Here's how the part is built. I have some questions about the finished solid (model axes, mm). A direction names the side the tool comes from. Coordinates: 2 decimals unless noted, no trailing zeros. Write each loop counter-clockwise with the first axis right and the second up, starting at its lowest first coordinate (ties: lowest second). Pieces come first, ordered by that corner, then holes. Notation, with made-up numbers: M -7,31.25 L 49,31.25 A19 cw 49,62.25 Z; hole C 65,87 d10. An arc over 180 degrees is marked long. Use one line per item in the form item = value. Start each with the question number.
1. Thinking about a two-plate mould opening in Y: for faces 1 (the face through (1, 0, 39)), 2 (the face through (1, 56, 80)), 3 (the face through (0.99, 93.74, 42.34)), which applies, released by +Y, released by -Y, zero draft, split by the parting line, or undercut?
2. On a 3-axis mill with a long thin cutter (end or side, diameter ignored), from which of +Z, -Z, +X, -X, +Y, -Y can I reach the whole of each face in a straight line? I mean faces 4 (the face through (0, 54, 39)), 5 (the face through (2, 54, 33)). Say none if no direction works.
3. I want a section at D-D, the plane z = 69.5. List the corners of the cut face in (x, y) for me, plus the area to 3 significant figures.
4. I want a section at C-C, the plane x = 1.2. Count the separate pieces of the cut face and the enclosed holes in it, plus the area to 3 significant figures.
5. I want a section at B-B, the plane z = 20. List the corners of the cut face in (x, y) for me, plus the area to 3 significant figures.
6. Please list where these lines run through material, in increasing order: line 1 along Y through (x, z) = (1.05, 20); line 2 along Z through (x, y) = (1.35, 92.5); line 3 along Y through (x, z) = (1.35, 73.5). Write a range as [from, to].
7. I'm going to push flat-ended pins straight in: pin 1 Ø3 at (y, z) = (40, 20) entering from -X; pin 2 Ø2 at (y, z) = (55, 28) entering from -X; pin 3 Ø6 at (y, z) = (56.5, 34) entering from +X. Where does each tip first touch, or does it pass through?
8. I want a section at A-A, the plane y = 55. List the corners of the cut face in (x, z) for me, plus the area to 3 significant figures.
from build123d import *

# Parameters (mm, degrees)
SKETCH1_W           = 155
SKETCH1_H           = 110
BOSS_EXTRUDE1_DEPTH = 80
SKETCH2_W           = 151
SKETCH2_H           = 106
CUT_EXTRUDE1_DEPTH  = 78
SKETCH3_R           = 2.5
CUT_EXTRUDE2_DEPTH  = 2
SKETCH7_R           = 1.6
CUT_EXTRUDE7_DEPTH  = 2
SKETCH4_W           = 27.5
SKETCH4_H           = 46.8
CUT_EXTRUDE8_DEPTH  = 2
SKETCH8_W           = 4
SKETCH8_H           = 53
CUT_EXTRUDE9_DEPTH  = 2
SKETCH9_W           = 14
SKETCH9_H           = 14
CUT_EXTRUDE10_DEPTH = 2
SKETCH10_W          = 25.2
SKETCH10_H          = 71.2
SKETCH10_R          = 1.25
CUT_EXTRUDE12_DEPTH = 2
SKETCH11_R          = 2.5
SKETCH11_R_2        = 4.5
CUT_EXTRUDE13_DEPTH = 2
SKETCH12_W          = 152.88518354
SKETCH12_H          = 110
CUT_EXTRUDE14_DEPTH = 80


with BuildPart() as part:
    # Sketch1 → Boss-Extrude1 (new body)
    with BuildSketch(Plane.XY):
        with Locations((77.5, 55)):
            Rectangle(SKETCH1_W, SKETCH1_H)
    extrude(amount=BOSS_EXTRUDE1_DEPTH)

    # Sketch2 → Cut-Extrude1 (cut)
    with BuildSketch(Plane.XY.offset(80)):
        with Locations((77.5, 55)):
            Rectangle(SKETCH2_W, SKETCH2_H)
    extrude(amount=-CUT_EXTRUDE1_DEPTH, mode=Mode.SUBTRACT)

    # Sketch3 → Cut-Extrude2 (cut)
    with BuildSketch(Plane.XY.offset(2)):
        with Locations((145, 100.5)):
            Circle(SKETCH3_R)
        with Locations((145, 9.5)):
            Circle(SKETCH3_R)
        with Locations((10, 9.5)):
            Circle(SKETCH3_R)
        with Locations((10, 100.5)):
            Circle(SKETCH3_R)
    extrude(amount=-CUT_EXTRUDE2_DEPTH, mode=Mode.SUBTRACT)

    # Sketch7 → Cut-Extrude7 (cut)
    with BuildSketch(Plane(origin=(0, 110, 0), x_dir=(1, 0, 0), z_dir=(0, 1, 0))):
        with Locations((44.48, -20.14450396)):
            Circle(SKETCH7_R)
        with Locations((95.28, -17.14)):
            Circle(SKETCH7_R)
        with Locations((95.28, -62.86)):
            Circle(SKETCH7_R)
        with Locations((44.48, -47.62)):
            Circle(SKETCH7_R)
    extrude(amount=-CUT_EXTRUDE7_DEPTH, mode=Mode.SUBTRACT)

    # Sketch4 → Cut-Extrude8 (cut)
    with BuildSketch(Plane(origin=(155, 0, 0), x_dir=(0, 0, -1), z_dir=(1, 0, 0))):
        with Locations((-40, 82.5)):
            Rectangle(SKETCH4_W, SKETCH4_H)
    extrude(amount=-CUT_EXTRUDE8_DEPTH, mode=Mode.SUBTRACT)

    # Sketch8 → Cut-Extrude9 (cut)
    with BuildSketch(Plane(origin=(155, 0, 0), x_dir=(0, 0, -1), z_dir=(1, 0, 0))):
        with Locations((-68, 28.5)):
            Rectangle(SKETCH8_W, SKETCH8_H)
        with Locations((-76, 28.5)):
            Rectangle(SKETCH8_W, SKETCH8_H)
        with Locations((-60, 28.5)):
            Rectangle(SKETCH8_W, SKETCH8_H)
        with Locations((-52, 28.5)):
            Rectangle(SKETCH8_W, SKETCH8_H)
        with Locations((-44, 28.5)):
            Rectangle(SKETCH8_W, SKETCH8_H)
        with Locations((-36, 28.5)):
            Rectangle(SKETCH8_W, SKETCH8_H)
        with Locations((-28, 28.5)):
            Rectangle(SKETCH8_W, SKETCH8_H)
        with Locations((-20, 28.5)):
            Rectangle(SKETCH8_W, SKETCH8_H)
        with Locations((-12, 28.5)):
            Rectangle(SKETCH8_W, SKETCH8_H)
        with Locations((-4, 28.5)):
            Rectangle(SKETCH8_W, SKETCH8_H)
    extrude(amount=-CUT_EXTRUDE9_DEPTH, mode=Mode.SUBTRACT)

    # Sketch9 → Cut-Extrude10 (cut)
    with BuildSketch(Plane(origin=(0, 110, 0), x_dir=(1, 0, 0), z_dir=(0, 1, 0))):
        with Locations((120, -19)):
            Rectangle(SKETCH9_W, SKETCH9_H)
    extrude(amount=-CUT_EXTRUDE10_DEPTH, mode=Mode.SUBTRACT)

    # Sketch10 → Cut-Extrude12 (cut)
    with BuildSketch(Plane.ZY):
        with Locations((58, 55)):
            Rectangle(SKETCH10_W, SKETCH10_H)
        with Locations((42.5, 92.5)):
            Circle(SKETCH10_R)
        with Locations((73.5, 92.5)):
            Circle(SKETCH10_R)
        with Locations((42.5, 17.5)):
            Circle(SKETCH10_R)
        with Locations((73.5, 17.5)):
            Circle(SKETCH10_R)
    extrude(amount=-CUT_EXTRUDE12_DEPTH, mode=Mode.SUBTRACT)

    # Sketch11 → Cut-Extrude13 (cut)
    with BuildSketch(Plane.ZY):
        with Locations((20, 55)):
            Circle(SKETCH11_R)
        with Locations((20, 40)):
            Circle(SKETCH11_R)
        with Locations((20, 25)):
            Circle(SKETCH11_R)
        with Locations((20, 82.5)):
            Circle(SKETCH11_R_2)
    extrude(amount=-CUT_EXTRUDE13_DEPTH, mode=Mode.SUBTRACT)

    # Sketch12 → Cut-Extrude14 (cut)
    with BuildSketch(Plane.XY.offset(80)):
        with Locations((78.55740823, 55)):
            Rectangle(SKETCH12_W, SKETCH12_H)
    extrude(amount=-CUT_EXTRUDE14_DEPTH, mode=Mode.SUBTRACT)


solid = part.part
Answer list:
q1.face_1 = released by -Y
q1.face_2 = zero draft
q1.face_3 = undercut
q2.face_4 = +Z, -Z, -X, +Y, -Y
q2.face_5 = +Z, +X
q3.outline = M 0,0 L 2.11,0 L 2.11,2 L 2,2 L 2,19.4 L 0,19.4 Z; M 0,90.6 L 2,90.6 L 2,108 L 2.11,108 L 2.11,110 L 0,110 Z
q3.area = 78.1 mm²
q4.separate_pieces = 1
q4.enclosed_holes = 9
q4.area = 6,860 mm²
q5.outline = M 0,0 L 2.11,0 L 2.11,2 L 2,2 L 2,22.5 L 0,22.5 Z; M 0,27.5 L 2,27.5 L 2,37.5 L 0,37.5 Z; M 0,42.5 L 2,42.5 L 2,52.5 L 0,52.5 Z; M 0,57.5 L 2,57.5 L 2,78 L 0,78 Z; M 0,87 L 2,87 L 2,108 L 2.11,108 L 2.11,110 L 0,110 Z
q5.area = 172 mm²
q6.line_1 = [0, 22.5], [27.5, 37.5], [42.5, 52.5], [57.5, 78], [87, 110]
q6.line_2 = [0, 41.25], [43.75, 72.25], [74.75, 80]
q6.line_3 = [0, 16.25], [18.75, 91.25], [93.75, 110]
q7.pin_1 = through
q7.pin_2 = 0
q7.pin_3 = 2
q8.outline = M 0,0 L 2.11,0 L 2.11,2 L 2,2 L 2,17.5 L 0,17.5 Z; M 0,22.5 L 2,22.5 L 2,45.4 L 0,45.4 Z; M 0,70.6 L 2,70.6 L 2,80 L 0,80 Z
q8.area = 99.8 mm²
